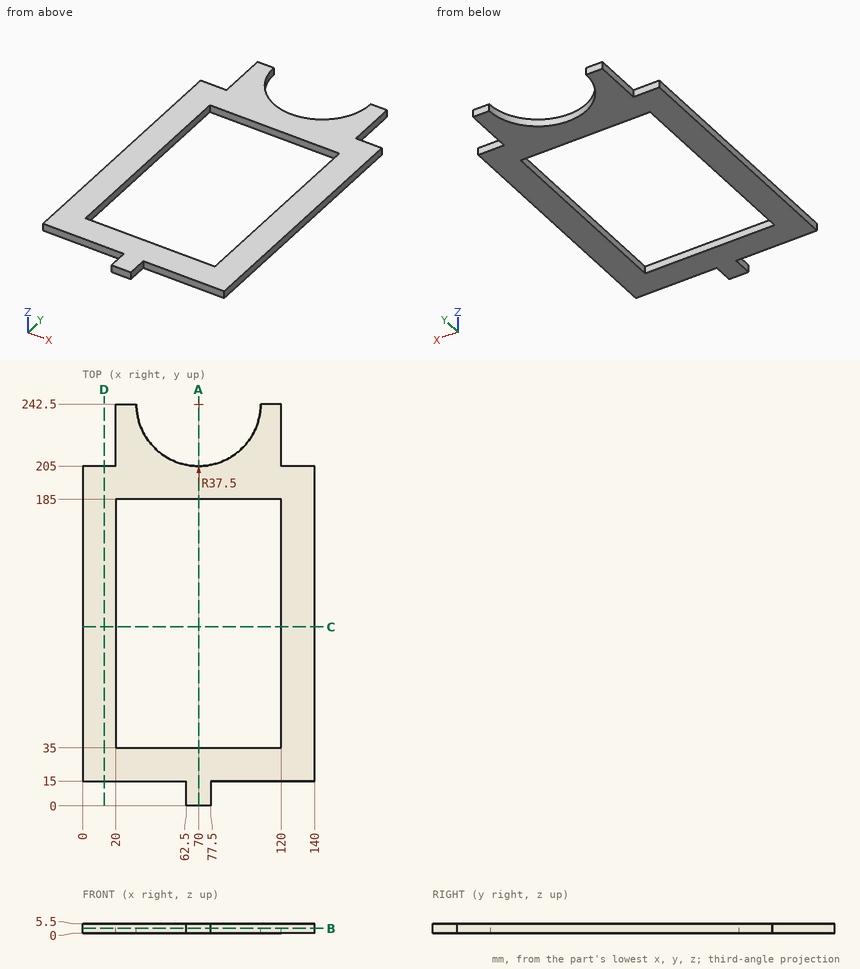
For this review, use the dimensioned drawing (mm, ordinates from the lowest corner) and the shaded views. Give positions to 0.01 mm unless a question says otherwise; leave off trailing zeros. Order: outer loops, then holes, each group sorted by start corner. A loop starts at its lowest first (then second) coordinate and runs counter-clockwise, first axis right, second up.
1) Take a section at A-A (x = 70). Give the boundary of the cut face in (y, z).
2) Insertion check: pin 1 (1.6 mm diameter, centred on y = 216, z = 2, fed in from -X); pin 2 (6 mm diameter, centred on x = 95, y = 180.5, fed in from -Z). Each pin has a flat end and moves straight along its axis. Give the tip position at first contact, or say it passes through.
3) Take a section at B-B (z = 2.8). Give the boundary of the cut face in (x, y), then the cut area to 3 significant figures.
4) Take a section at C-C (y = 108). Give the boundary of the cut face in (x, z), then the cut area to 3 significant figures.
5) Take a section at D-D (x = 13). Give the boundary of the cut face in (y, z), then the cut area to 4 significant figures.
6) Wall thickness on line 1 (X direction, y = 150, z = 4.25); line 2 (Y direction, x = 43, z = 0.7); line 3 (Y direction, x = 87, z = 3.1): over which ranges is each line inside the solid? List them lowest first.
Derived:
1. outline: (0, 0) - (35, 0) - (35, 5.5) - (0, 5.5) - close; (185, 0) - (205, 0) - (205, 5.5) - (185, 5.5) - close
2. pin 1: stops at x = 20
2. pin 2: passes through
3. outline: (0, 15) - (62.5, 15) - (62.5, 0) - (77.5, 0) - (77.5, 15) - (140, 15) - (140, 205) - (120, 205) - (120, 242.5) - (107.5, 242.5) arc R37.5 cw to (32.5, 242.5) - (20, 242.5) - (20, 205) - (0, 205) - close; hole (20, 35) - (120, 35) - (120, 185) - (20, 185) - close
3. area: 13,400 mm2
4. outline: (0, 0) - (20, 0) - (20, 5.5) - (0, 5.5) - close; (120, 0) - (140, 0) - (140, 5.5) - (120, 5.5) - close
4. area: 220 mm2
5. outline: (15, 0) - (205, 0) - (205, 5.5) - (15, 5.5) - close
5. area: 1,045 mm2
6. line 1: x = 0 to 20, 120 to 140
6. line 2: y = 15 to 35, 185 to 216.48
6. line 3: y = 15 to 35, 185 to 209.07
